The drawing under review shows one solid part. Ordinate dimensions are in mm from its lowest x, y, z. Round coordinates to 2 decimals unless told otherwise and drop trailing zeros. Write each loop counter-clockwise with the first axis right and the second up, starting at its lowest first coordinate (ties: lowest second). Pieces come first, ordered by that corner, then holes. Notation, with made-up numbers: (48.25, 88.5) -> (89.25, 88.5) arc R29 ccw to (89.25, 119.5) -> close; hole circle Ø2 at (-7.5, 84). An arc over 180 degrees is marked (long way). Use CSV: the item, a comma, the result in double quotes. Start each with the question number.
1) Take a section at A-A, the plane y = 24. Give the boundary of the cut face in (x, z).
2) Take a section at B-B, the plane x = 26. Give the boundary of the cut face in (y, z).
3) Wall thickness on probe 1 along Y at (x, z) = (31.5, 0.6); probe 2 along X at (y, z) = (25.5, 0.85): over which ranges is each line inside the solid? List them lowest first. Write a range as [from, to].
4) Take a section at C-C, the plane z = 0.6. Give the boundary of the cut face in (x, y), then the cut area to 3 significant figures.
5) For pin 1 Ø8 at (x, y) = (16.5, 17) entering from +Z, flat-tipped, find the tip position at first contact; note if it passes through.
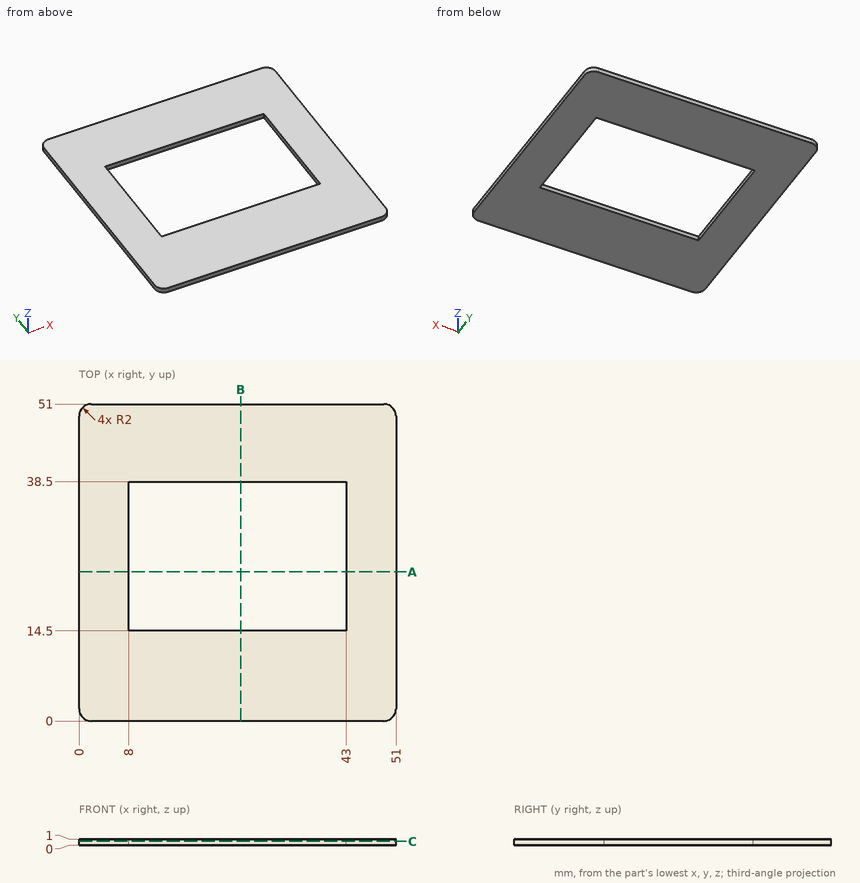
Values found:
1,outline,"(0, 0) -> (8, 0) -> (8, 1) -> (0, 1) -> close; (43, 0) -> (51, 0) -> (51, 1) -> (43, 1) -> close"
2,outline,"(0, 0) -> (14.5, 0) -> (14.5, 1) -> (0, 1) -> close; (38.5, 0) -> (51, 0) -> (51, 1) -> (38.5, 1) -> close"
3,probe 1,"[0, 14.5], [38.5, 51]"
3,probe 2,"[0, 8], [43, 51]"
4,outline,"(0, 2) arc R2 ccw to (2, 0) -> (49, 0) arc R2 ccw to (51, 2) -> (51, 49) arc R2 ccw to (49, 51) -> (2, 51) arc R2 ccw to (0, 49) -> close; hole (8, 14.5) -> (43, 14.5) -> (43, 38.5) -> (8, 38.5) -> close"
4,area,"1,760 mm²"
5,pin 1,"z = 1"
